Here's how the part is built. I have some questions about the finished solid (model axes, mm). Face numbers are marked on the shaded views. A direction names the side the tool comes from. Coordinates: 2 decimals unless noted, no trailing zeros. Loops run counter-clockwise (first coordinate to the right, second up) from the corner with the lowest first, then second, coordinate; pieces in that order, holes last. Notation, with made-up numbers: (58.5, 39) -> (113.5, 39) arc R11 ccw to (113.5, 45) -> close; hole circle Ø4 at (50.5, 81.5). An arc over 180 degrees is marked (long way). Answer as a JSON object with one key per item and string values. Group by question number.
Q1. I want a section at B-B on x = -17. Count the separate pieces of the cut face and the enclosed holes in it, then the cut area to 3 significant figures.
Q2. On a 3-axis mill with a long thin cutter (end or side, diameter ignored), from which of +Z, -Z, +X, -X, +Y, -Y can I reach the whole of each face in a straight line? I mean the marked faces 3, 4 and 5. Say none if no direction works.
Q3. Thinking about a two-plate mould opening in Z: for the marked faces 1 and 2, which applies, released by +Z, released by -Z, zero draft, split by the parting line, or undercut?
Q4. I'm going to push flat-ended pins straight in: pin 1 (6.5 mm diameter, centred on x = -3, z = -2, fed in from +Y); pin 2 (1.6 mm diameter, centred on y = 1, z = -1, fed in from +X); pin 3 (1 mm diameter, centred on y = 1.5, z = -1.5, fed in from -X). Where does each tip first touch, or does it pass through?
Q5. I need wall thicknesses on line 1 (Z direction, x = 9, y = 1.35); line 2 (Z direction, x = 13, y = -0.95); line 3 (X direction, y = -0.25, z = -16). Which ranges of each line are inside material? Lowest first, please.
Q6. I want a section at A-A on z = 0. Write out the boundary of the cut face in (x, y) (3 decimals), then the cut area to 3 significant figures.
```python
from build123d import *

# Parameters (mm, degrees)
CUT_EXTRUDE1_DEPTH = 41.519966486
CIRPATTERN1_COUNT  = 4
CUT_EXTRUDE2_DEPTH = 2.032
SKETCH7_R          = 2.413
CUT_EXTRUDE3_DEPTH = 41.519966486


with BuildPart() as part:
    # Sketch1 → Revolve1 (revolve)
    with BuildSketch(Plane(origin=(0, 0, 0), x_dir=(0, 0, -1), z_dir=(1, 0, 0)), mode=Mode.PRIVATE) as revolve1_sk:
        with BuildLine():
            Line((0, -1.651), (0, 1.651))
            Line((0, 1.651), (0, 2.413))
            Line((0, 2.413), (-28.448, 2.413))
            Line((-28.448, 2.413), (-28.448, 1.651))
            ThreePointArc((-28.448, 1.651), (-26.797, 0), (-28.448, -1.651))
            Line((-28.448, -1.651), (-28.448, -2.413))
            Line((-28.448, -2.413), (0, -2.413))
            Line((0, -2.413), (0, -1.651))
        make_face()
    revolve(revolve1_sk.sketch.rotate(Axis((0, -1.651, 0), (0, 1, 0)), 180), axis=Axis((0, -1.651, 0), (0, 1, 0)))

    # Sketch4 → Cut-Extrude1 (cut, through all)
    with BuildSketch(Plane(origin=(0, 2.413, 0), x_dir=(1, 0, 0), z_dir=(0, 1, 0))):
        with BuildLine():
            Line((-18.150933962, -3.200499383), (-13.725620051, -2.420197142))
            ThreePointArc((-13.725620051, -2.420197142), (-11.215481947, -2.795189817), (-9.436261178, -4.605103146))
            ThreePointArc((-9.436261178, -4.605103146), (-7.424621202, -7.424621202), (-4.605103146, -9.436261178))
            ThreePointArc((-4.605103146, -9.436261178), (-2.795189817, -11.215481947), (-2.420197142, -13.725620051))
            Line((-2.420197142, -13.725620051), (-3.200499383, -18.150933962))
            ThreePointArc((-3.200499383, -18.150933962), (-5.207970247, -20.958954952), (-8.653989227, -21.158640563))
            ThreePointArc((-8.653989227, -21.158640563), (-16.164461018, -16.164461018), (-21.158640563, -8.653989227))
            ThreePointArc((-21.158640563, -8.653989227), (-20.958954952, -5.207970247), (-18.150933962, -3.200499383))
        make_face()
    cut_extrude1 = extrude(amount=-CUT_EXTRUDE1_DEPTH, mode=Mode.SUBTRACT)

    # CirPattern1: Cut-Extrude1 ×4 about axis
    cirpattern1_axis = Axis((0, 0, 0), (0, 1, 0))
    for i in range(1, CIRPATTERN1_COUNT):
        add(cut_extrude1.rotate(cirpattern1_axis, i * 360 / CIRPATTERN1_COUNT), mode=Mode.SUBTRACT)

    # Sketch6 → Cut-Extrude2 (cut)
    with BuildSketch(Plane(origin=(0, 2.413, 0), x_dir=(1, 0, 0), z_dir=(0, 1, 0))):
        Polygon((0, 7.661438072), (-6.635, 3.830719036), (-6.635, -3.830719036), (0, -7.661438072), (6.635, -3.830719036), (6.635, 3.830719036), align=None)
    extrude(amount=-CUT_EXTRUDE2_DEPTH, mode=Mode.SUBTRACT)

    # Sketch7 → Cut-Extrude3 (cut, through all)
    with BuildSketch(Plane(origin=(0, 2.413, 0), x_dir=(1, 0, 0), z_dir=(0, 1, 0))):
        with Locations(Location((0, 0, 0), (0, 0, 270))):
            Circle(SKETCH7_R)
    extrude(amount=-CUT_EXTRUDE3_DEPTH, mode=Mode.SUBTRACT)


solid = part.part
```
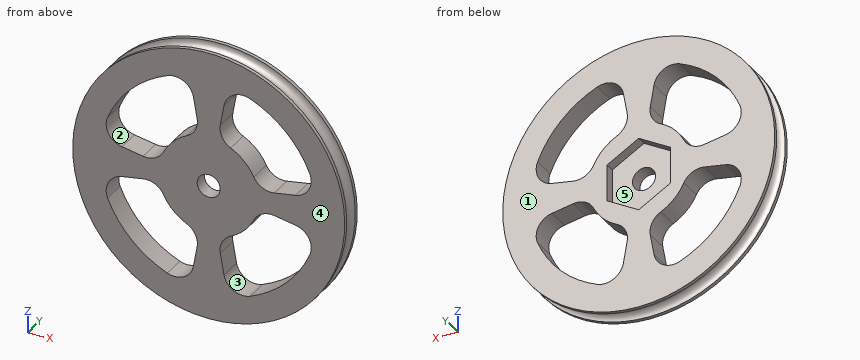
Result set:
{
 "1": {"separate pieces": "3", "enclosed holes": "0", "area": "90.7 mm²"},
 "2": {"face 3": "+Y, -Y", "face 4": "+Z, -Z, +X, -X, -Y", "face 5": "+Y"},
 "3": {"face 1": "zero draft", "face 2": "undercut"},
 "4": {"pin 1": "stops at y = 0.38", "pin 2": "stops at x = 28.44", "pin 3": "stops at x = -28.43"},
 "5": {"line 1": "z = -25.98 to -21.01, -5.41 to 5.41, 21.01 to 25.98", "line 2": "z = -23.78 to -18.8, -2.36 to 2.36, 18.8 to 23.78", "line 3": "x = -21.52 to -16.33, -2.82 to 2.82, 16.33 to 21.52"},
 "6": {"outline": "(-28.448, -2.413) -> (-2.413, -2.413) -> (-2.413, 0.381) -> (-6.635, 0.381) -> (-6.635, 2.413) -> (-28.448, 2.413) -> (-28.448, 1.651) arc R1.651 cw to (-28.448, -1.651) -> close; (2.413, -2.413) -> (28.448, -2.413) -> (28.448, -1.651) arc R1.651 cw to (28.448, 1.651) -> (28.448, 2.413) -> (6.635, 2.413) -> (6.635, 0.381) -> (2.413, 0.381) -> close", "area": "226 mm²"}
}
